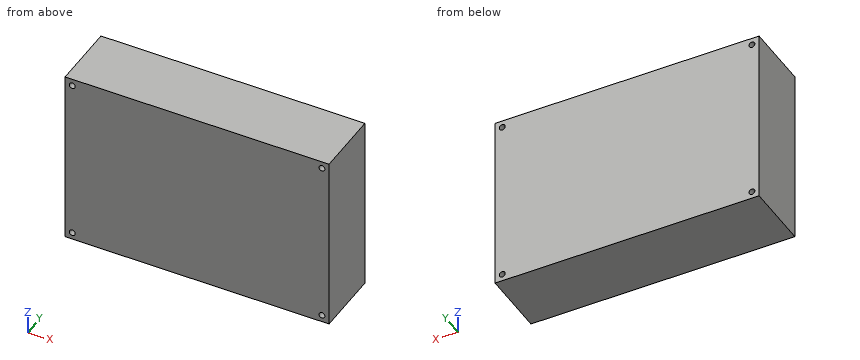
from build123d import *

# Parameters (mm, degrees)
SKETCH_1_W      = 93.98
SKETCH_1_H      = 63.5
SKETCH_1_R      = 1.05
EXTRUDE_1_DEPTH = 1.7
EXTRUDE_START   = 1.7
SKETCH_1_4_W    = 93.98
SKETCH_1_4_H    = 63.5
SKETCH_1_4_R    = 1.05
EXTRUDE_2_DEPTH = 22


with BuildPart() as part:
    # 草图1 → 凸台-拉伸1 (new body)
    with BuildSketch(Plane(origin=(0, 0, 0), x_dir=(1, 0, 0), z_dir=(0, 1, 0))):
        Rectangle(SKETCH_1_W, SKETCH_1_H)
        with Locations(Location((-44.45, 29.21, 0), (0, 0, 270))):
            Circle(SKETCH_1_R, mode=Mode.SUBTRACT)
        with Locations(Location((-44.45, -29.21, 0), (0, 0, 270))):
            Circle(SKETCH_1_R, mode=Mode.SUBTRACT)
        with Locations(Location((44.45, 29.21, 0), (0, 0, 270))):
            Circle(SKETCH_1_R, mode=Mode.SUBTRACT)
        with Locations(Location((44.45, -29.21, 0), (0, 0, 270))):
            Circle(SKETCH_1_R, mode=Mode.SUBTRACT)
    extrude(amount=EXTRUDE_1_DEPTH)

    # 草图1<4> → 凸台-拉伸2 (add)
    with BuildSketch(Plane(origin=(0, 0, 0), x_dir=(1, 0, 0), z_dir=(0, 1, 0)).offset(EXTRUDE_START)):
        Rectangle(SKETCH_1_4_W, SKETCH_1_4_H)
        with Locations(Location((-44.45, 29.21, 0), (0, 0, 90))):
            Circle(SKETCH_1_4_R, mode=Mode.SUBTRACT)
        with Locations(Location((-44.45, -29.21, 0), (0, 0, 90))):
            Circle(SKETCH_1_4_R, mode=Mode.SUBTRACT)
        with Locations(Location((44.45, 29.21, 0), (0, 0, 90))):
            Circle(SKETCH_1_4_R, mode=Mode.SUBTRACT)
        with Locations(Location((44.45, -29.21, 0), (0, 0, 90))):
            Circle(SKETCH_1_4_R, mode=Mode.SUBTRACT)
    extrude(amount=EXTRUDE_2_DEPTH)


solid = part.part
Work out the finished part from the listing and answer in its coordinate system (mm). Round coordinates to 2 decimals unless told otherwise and drop trailing zeros. Loops run counter-clockwise (first coordinate to the right, second up) from the corner with the lowest first, then second, coordinate; pieces in that order, holes last. Notation, with made-up numbers: M 59,63.5 L 116,63.5 A27 ccw 116,81.5 Z; hole C -28.5,5 d10. An arc over 180 degrees is marked long. One line per question, with ' | ' between items. Start each with the question number.
(1) A cutting plane is placed at B-B on z = -29.21. Write down the section's boundary in (x, y).
(2) Find the intervals of material crossed by line 1 (X direction, y = 9, z = 29.21); line 2 (Z direction, x = -44.45, y = 18.5), in increasing order.
(3) A cutting plane is placed at A-A on x = 44.45. Write down the section's boundary in (y, z), plus the area to 3 significant figures.
Geometry check:
1) outline: M -46.99,0 L -45.5,0 L -45.5,23.7 L -46.99,23.7 Z; M -43.4,0 L 43.4,0 L 43.4,23.7 L -43.4,23.7 Z; M 45.5,0 L 46.99,0 L 46.99,23.7 L 45.5,23.7 Z
2) line 1: x = -46.99 to -45.5, -43.4 to 43.4, 45.5 to 46.99 | line 2: z = -31.75 to -30.26, -28.16 to 28.16, 30.26 to 31.75
3) outline: M 0,-31.75 L 23.7,-31.75 L 23.7,-30.26 L 0,-30.26 Z; M 0,-28.16 L 23.7,-28.16 L 23.7,28.16 L 0,28.16 Z; M 0,30.26 L 23.7,30.26 L 23.7,31.75 L 0,31.75 Z | area: 1,410 mm²
